Design review of the part built by this model. Coordinates are the model's own, in mm. Face numbers are marked on the shaded views. A direction names the side the tool comes from. Coordinates: 2 decimals unless noted, no trailing zeros. Write each loop counter-clockwise with the first axis right and the second up, starting at its lowest first coordinate (ties: lowest second). Pieces come first, ordered by that corner, then holes.
Q1. Clearance check with a flat-ended pin moving along its axis: pin 1 Ø6.5 at (y, z) = (-9, 17) entering from +X. State where the tip first meets the part, or that it passes through.
Q2. The part is to be moulded in two halves that separate along Z. For the marked faces 1, 2, 3 and 4, say which applies: +Z half, -Z half, draft (parallel to the pull), parting line (faces both ways), or undercut.
Q3. Add section A-A, the plane x = 12.7. Give the boundary of the cut face in (y, z).
Q4. Add section D-D, the plane y = 7.75. Give the boundary of the cut face in (x, z), plus the area to 3 significant figures.
Q5. Add section C-C, the plane y = -8.75. Give the boundary of the cut face in (x, z), plus the area to 3 significant figures.
Q6. Add section B-B, the plane z = 14.25. Give the boundary of the cut face in (x, y), plus the area to 3 significant figures.
Q7. Machinability: for the marked faces 5, 6 and 7, which of the approach directions +Z, -Z, +X, -X, +Y, -Y give a long, thin tool a straight path to every point of the face, cutting with its end or side? Answer none if there is none.
Q8. To check wall thickness, follow probe 1 along Z at (x, y) = (12.7, 8); probe 2 along Y at (x, z) = (10.5, 4.25); probe 3 along X at (y, z) = (-1.25, 3.25). State the ranges of each line that lie inside material, in increasing order.
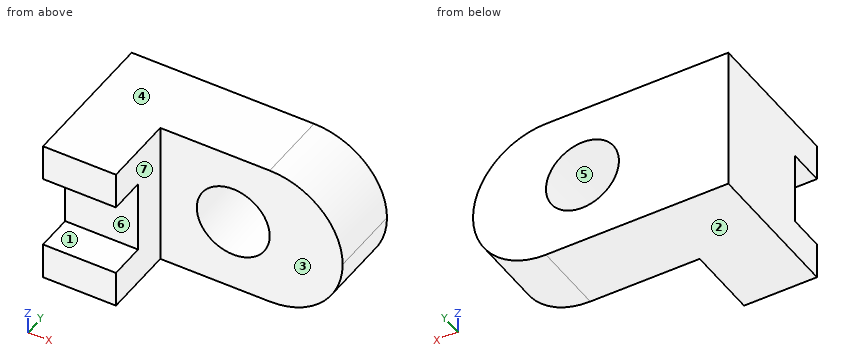
from build123d import *

# Parameters (mm, degrees)
F1_DEPTH = 25.4
F2_W     = 12.7
F2_H     = 12.7
F3_DEPTH = 6.35
F5_DEPTH = 25.4
F6_R     = 6.35
F7_DEPTH = 25.4


with BuildPart() as f1:
    # F0 (on Top) → F1 (new body)
    with BuildSketch(Plane.XY):
        Polygon((0, -12.7), (0, 0), (31.75, 0), (31.75, 12.7), (-12.7, 12.7), (-12.7, -12.7), align=None)
    extrude(amount=F1_DEPTH)

    # F2 (on face) → F3 (cut)
    with BuildSketch(Plane.XZ.offset(12.7)):
        with Locations((-6.35, 12.7)):
            Rectangle(F2_W, F2_H)
    extrude(amount=-F3_DEPTH, mode=Mode.SUBTRACT)

    # F4 (on face) → F5 (cut)
    with BuildSketch(Plane.XZ):
        with BuildLine():
            ThreePointArc((19.05, 25.4), (28.030256, 21.680256), (31.75, 12.7))
            Line((31.75, 12.7), (31.75, 25.4))
            Line((31.75, 25.4), (19.05, 25.4))
        make_face()
        with BuildLine():
            ThreePointArc((31.75, 12.7), (28.030256, 3.719744), (19.05, 0))
            Line((19.05, 0), (31.75, 0))
            Line((31.75, 0), (31.75, 12.7))
        make_face()
    extrude(amount=-F5_DEPTH, mode=Mode.SUBTRACT)

    # F6 (on face) → F7 (cut)
    with BuildSketch(Plane.XZ):
        with Locations((12.7, 12.7)):
            Circle(F6_R)
    extrude(amount=-F7_DEPTH, mode=Mode.SUBTRACT)


solid = f1.part
Here are the results:
1. pin 1: stops at x = 0
2. face 1: undercut
2. face 2: -Z half
2. face 3: draft
2. face 4: +Z half
3. outline: (0, 0) - (12.7, 0) - (12.7, 6.35) - (0, 6.35) - close; (0, 19.05) - (12.7, 19.05) - (12.7, 25.4) - (0, 25.4) - close
4. outline: (-12.7, 0) - (19.05, 0) arc R12.7 ccw to (19.05, 25.4) - (-12.7, 25.4) - close; hole circle Ø12.7 at (12.7, 12.7)
4. area: 933 mm2
5. outline: (-12.7, 0) - (0, 0) - (0, 6.35) - (-12.7, 6.35) - close; (-12.7, 19.05) - (0, 19.05) - (0, 25.4) - (-12.7, 25.4) - close
5. area: 161 mm2
6. outline: (-12.7, -6.35) - (0, -6.35) - (0, 0) - (6.54, 0) - (6.54, 12.7) - (-12.7, 12.7) - close; (18.86, 0) - (31.66, 0) - (31.66, 12.7) - (18.86, 12.7) - close
6. area: 488 mm2
7. face 5: +Y, -Y
7. face 6: +X, -X, -Y
7. face 7: +Z, -Z, +X, -Y
8. probe 1: z = 0 to 6.35, 19.05 to 25.4
8. probe 2: y = 0 to 12.7
8. probe 3: x = -12.7 to 0
